from build123d import *

# Parameters (mm, degrees)
SKETCH1_R                       = 48.5
SKETCH1_R_2                     = 1.5
BOSS_EXTRUDE1_DEPTH             = 4
SKETCH2_R                       = 3.75
CUT_EXTRUDE1_DEPTH              = 1.5
BOSS_EXTRUDE2_START             = 4
SKETCH3_R                       = 9
BOSS_EXTRUDE2_DEPTH             = 14
CUT_EXTRUDE3_START              = 6
SKETCH4_R                       = 1.3
CUT_EXTRUDE3_DEPTH              = 91.444646155
BOSS_EXTRUDE3_DEPTH             = 9
BOSS_EXTRUDE3_DIRECTION_2_REACH = 108.638
CUT_EXTRUDE4_DEPTH              = 101.75311462
CUT_EXTRUDE4_DEPTH_BACK         = 101.75311462
FILLET1_R                       = 10
FILLET2_R                       = 2


with BuildPart() as part:
    # Sketch1 → Boss-Extrude1 (new body)
    with BuildSketch(Plane(origin=(0, 0, 0), x_dir=(1, 0, 0), z_dir=(0, 1, 0))):
        with Locations(Location((0, 0, 0), (0, 0, 270))):
            Circle(SKETCH1_R)
        with Locations(Location((0, 7.25, 0), (0, 0, 270))):
            Circle(SKETCH1_R_2, mode=Mode.SUBTRACT)
        with Locations(Location((0, -7.25, 0), (0, 0, 270))):
            Circle(SKETCH1_R_2, mode=Mode.SUBTRACT)
    extrude(amount=BOSS_EXTRUDE1_DEPTH)

    # Sketch2 → Cut-Extrude1 (cut)
    with BuildSketch(Plane.XZ):
        with Locations(Location((0, 0, 0), (0, 0, 270))):
            Circle(SKETCH2_R)
    extrude(amount=-CUT_EXTRUDE1_DEPTH, mode=Mode.SUBTRACT)

    # Sketch3 → Boss-Extrude2 (add)
    with BuildSketch(Plane(origin=(0, 0, 0), x_dir=(0, 0, -1), z_dir=(1, 0, 0)).offset(BOSS_EXTRUDE2_START)):
        with BuildLine():
            Line((30.34, 4), (-30.34, 4))
            Line((-30.34, 4), (-30.34, 11.86))
            ThreePointArc((-30.34, 11.86), (-28.924736696, 21.745164753), (-24.792654999, 30.836113728))
            Line((-24.792654999, 30.836113728), (-9.278105641, 55.104149989))
            ThreePointArc((-9.278105641, 55.104149989), (30.651097233, 62.12443475), (34.252718415, 21.743078098))
            ThreePointArc((34.252718415, 21.743078098), (31.352340729, 17.057138369), (30.34, 11.64))
            Line((30.34, 11.64), (30.34, 4))
        make_face()
        with Locations((13.91, 40.28)):
            Circle(SKETCH3_R, mode=Mode.SUBTRACT)
    extrude(amount=BOSS_EXTRUDE2_DEPTH)

    # Sketch4 → Cut-Extrude3 (cut, through all)
    with BuildSketch(Plane(origin=(0, 0, 0), x_dir=(0, 0, -1), z_dir=(1, 0, 0)).offset(CUT_EXTRUDE3_START)):
        Polygon((-15.259242405, 25.959242405), (13.732135624, 54.950620434), (28.581378029, 40.101378029), (-0.41, 11.11), align=None)
        with Locations(Location((-13.845028843, 19.595281374, 0), (0, 0, 180))):
            Circle(SKETCH4_R)
        with Locations(Location((-6.773961031, 12.524213562, 0), (0, 0, 180))):
            Circle(SKETCH4_R)
        with Locations(Location((20.096096654, 53.536406871, 0), (0, 0, 180))):
            Circle(SKETCH4_R)
        with Locations(Location((27.167164466, 46.465339059, 0), (0, 0, 180))):
            Circle(SKETCH4_R)
    extrude(amount=CUT_EXTRUDE3_DEPTH, mode=Mode.SUBTRACT)

    # Sketch5 → Boss-Extrude3 (add)
    with BuildSketch(Plane(origin=(18, 0, 0), x_dir=(0, 0, -1), z_dir=(1, 0, 0))):
        with BuildLine():
            Line((30.34, 4), (36.34, 4))
            Line((36.34, 4), (36.34, 11.64))
            ThreePointArc((36.34, 11.64), (36.947404437, 14.890283021), (38.687631049, 17.701846859))
            ThreePointArc((38.687631049, 17.701846859), (34.300821036, 66.886736311), (-14.333340667, 58.335960445))
            Line((-14.333340667, 58.335960445), (-29.847890025, 34.067924184))
            ThreePointArc((-29.847890025, 34.067924184), (-34.683704058, 23.428701186), (-36.34, 11.86))
            Line((-36.34, 11.86), (-36.34, 4))
            Line((-36.34, 4), (-30.34, 4))
            Line((-30.34, 4), (-30.34, 11.86))
            ThreePointArc((-30.34, 11.86), (-28.924736696, 21.745164753), (-24.792654999, 30.836113728))
            Line((-24.792654999, 30.836113728), (-14.162524076, 47.463886585))
            ThreePointArc((-14.162524076, 47.463886585), (-11.806963139, 51.339412511), (-9.278105641, 55.104149989))
            ThreePointArc((-9.278105641, 55.104149989), (30.651097233, 62.12443475), (34.252718415, 21.743078098))
            ThreePointArc((34.252718415, 21.743078098), (31.352340729, 17.057138369), (30.34, 11.64))
            Line((30.34, 11.64), (30.34, 4))
        make_face()
    extrude(amount=BOSS_EXTRUDE3_DEPTH)

    # Boss-Extrude3 direction 2: up to this face of the body (flat: up to its plane)
    boss_extrude3_direction_2_end = Plane(part.part.faces().sort_by_distance((4, 32.000889593, -6.762869766))[0])
    # Sketch5 → Boss-Extrude3 direction 2 (add, up to the picked face)
    with BuildSketch(Plane(origin=(18, 0, 0), x_dir=(0, 0, -1), z_dir=(1, 0, 0)), mode=Mode.PRIVATE) as boss_extrude3_direction_2_sk1:
        with BuildLine():
            Line((30.34, 4), (36.34, 4))
            Line((36.34, 4), (36.34, 11.64))
            ThreePointArc((36.34, 11.64), (36.947404437, 14.890283021), (38.687631049, 17.701846859))
            ThreePointArc((38.687631049, 17.701846859), (34.300821036, 66.886736311), (-14.333340667, 58.335960445))
            Line((-14.333340667, 58.335960445), (-29.847890025, 34.067924184))
            ThreePointArc((-29.847890025, 34.067924184), (-34.683704058, 23.428701186), (-36.34, 11.86))
            Line((-36.34, 11.86), (-36.34, 4))
            Line((-36.34, 4), (-30.34, 4))
            Line((-30.34, 4), (-30.34, 11.86))
            ThreePointArc((-30.34, 11.86), (-28.924736696, 21.745164753), (-24.792654999, 30.836113728))
            Line((-24.792654999, 30.836113728), (-14.162524076, 47.463886585))
            ThreePointArc((-14.162524076, 47.463886585), (-11.806963139, 51.339412511), (-9.278105641, 55.104149989))
            ThreePointArc((-9.278105641, 55.104149989), (30.651097233, 62.12443475), (34.252718415, 21.743078098))
            ThreePointArc((34.252718415, 21.743078098), (31.352340729, 17.057138369), (30.34, 11.64))
            Line((30.34, 11.64), (30.34, 4))
        make_face()
    boss_extrude3_direction_2_tool1 = split(extrude(boss_extrude3_direction_2_sk1.sketch, amount=-BOSS_EXTRUDE3_DIRECTION_2_REACH, mode=Mode.PRIVATE), bisect_by=boss_extrude3_direction_2_end, keep=Keep.BOTH, mode=Mode.PRIVATE)
    add(boss_extrude3_direction_2_tool1.solids().sort_by(Axis((18, 7.82, -31.430412), (-1, 0, 0)))[0])

    # Sketch6 → Cut-Extrude4 (cut, two sides: drawn at the far end of the back side and taken through both)
    with BuildSketch(Plane.XY.offset(-CUT_EXTRUDE4_DEPTH_BACK)):
        with BuildLine():
            Line((27, 73.801694463), (21, 73.801694463))
            ThreePointArc((21, 73.801694463), (22.52665425, 38.804454133), (26.5, 4))
            Line((26.5, 4), (27, 4))
            Line((27, 4), (27, 73.801694463))
        make_face()
    extrude(amount=CUT_EXTRUDE4_DEPTH + CUT_EXTRUDE4_DEPTH_BACK, mode=Mode.SUBTRACT)

    # Fillet1
    # the kernel refuses this fillet: 10 mm, written as the material it takes off along each edge
    with BuildSketch(Plane(origin=(4, 11.86, 36.34), x_dir=(0, 0, -1), z_dir=(0, -1, 0))) as fillet1_piece_1:
        with BuildLine():
            CenterArc((FILLET1_R, FILLET1_R), FILLET1_R, 180, 90)
            Line((0, FILLET1_R), (0, 0))
            Line((0, 0), (FILLET1_R, 0))
        make_face()
    extrude(amount=7.86, mode=Mode.SUBTRACT)
    with BuildSketch(Plane(origin=(4, 11.86, -4.89), x_dir=(0, 0.5386350760234976, 0.8425391711233141), z_dir=(0, 0.8425391711233141, -0.5386350760234976))) as fillet1_piece_2:
        with BuildLine():
            CenterArc((41.23 - FILLET1_R, FILLET1_R), FILLET1_R, 270, 90)
            Line((41.23, FILLET1_R), (41.23, 0))
            Line((41.23, 0), (41.23 - FILLET1_R, 0))
        make_face()
    revolve(axis=Axis((4, 11.86, -4.89), (1, 0, 0)), revolution_arc=32.590770812, mode=Mode.SUBTRACT)
    with BuildSketch(Plane(origin=(4, 58.335960445, 14.333340667), x_dir=(0, -0.5386350760234987, -0.8425391711233132), z_dir=(0, -0.8425391711233133, 0.5386350760234988))) as fillet1_piece_3:
        with BuildLine():
            CenterArc((FILLET1_R, FILLET1_R), FILLET1_R, 180, 90)
            Line((0, FILLET1_R), (0, 0))
            Line((0, 0), (FILLET1_R, 0))
        make_face()
    extrude(amount=28.803451629, mode=Mode.SUBTRACT)
    with BuildSketch(Plane(origin=(4, 40.28, -13.91), x_dir=(0, -0.6735385398377844, -0.7391521056948869), z_dir=(0, -0.7391521056948869, 0.6735385398377844))) as fillet1_piece_4:
        with BuildLine():
            CenterArc((33.521694463 - FILLET1_R, FILLET1_R), FILLET1_R, 270, 90)
            Line((33.521694463, FILLET1_R), (33.521694463, 0))
            Line((33.521694463, 0), (33.521694463 - FILLET1_R, 0))
        make_face()
    revolve(axis=Axis((4, 40.28, -13.91), (1, 0, 0)), revolution_arc=189.749991197, mode=Mode.SUBTRACT)
    with BuildSketch(Plane(origin=(4, 4, -36.34), x_dir=(0, 0, 1), z_dir=(0, 1, 0))) as fillet1_piece_5:
        with BuildLine():
            CenterArc((FILLET1_R, FILLET1_R), FILLET1_R, 180, 90)
            Line((0, FILLET1_R), (0, 0))
            Line((0, 0), (FILLET1_R, 0))
        make_face()
    extrude(amount=7.64, mode=Mode.SUBTRACT)
    with BuildSketch(Plane(origin=(4, 11.64, -45.34), x_dir=(0, 0.6735385398377856, 0.7391521056948859), z_dir=(0, 0.7391521056948859, -0.6735385398377856))) as fillet1_piece_6:
        with BuildLine():
            CenterArc((9 + FILLET1_R, FILLET1_R), FILLET1_R, 180, 90)
            Line((9, FILLET1_R), (9, 0))
            Line((9, 0), (9 + FILLET1_R, 0))
        make_face()
    revolve(axis=Axis((4, 11.64, -45.34), (1, 0, 0)), revolution_arc=42.340762009, mode=Mode.SUBTRACT)

    # Fillet2
    fillet2_edges = [part.edges().sort_by_distance(p)[0] for p in [
        (20.25, 4, -36.34),
        (20.25, 4, 36.34),
        (6.928932188, 4, 33.411067812),
        (4, 4, 0),
        (6.928932188, 4, -33.411067812),
    ]]
    fillet(fillet2_edges, radius=FILLET2_R)
    fillet2_2_edges = [part.edges().sort_by_distance(p)[0] for p in [
        (26.5, 4, -33.34),
    ]]
    fillet(fillet2_2_edges, radius=FILLET2_R)
    fillet2_3_edges = [part.edges().sort_by_distance(p)[0] for p in [
        (26.5, 4, 33.34),
    ]]
    fillet(fillet2_3_edges, radius=FILLET2_R)


solid = part.part
For this review, take the finished solid that the model builds, in its own axes (mm). A direction names the side the tool comes from. Give positions to 0.01 mm unless a question says otherwise; leave off trailing zeros. Loops run counter-clockwise (first coordinate to the right, second up) from the corner with the lowest first, then second, coordinate; pieces in that order, holes last.
Item 1: Take a section at A-A, the plane z = -7.25. Give the number of separate pieces and of enclosed holes in the cut face, and give its area (3 significant figures).
Item 2: Take a section at C-C, the plane x = -15. State the section outline as (y, z) points.
Item 3: Insertion check: pin 1 (4 mm diameter, centred on y = 55, z = 11, fed in from +X); pin 2 (6 mm diameter, centred on y = 50, z = -37.5, fed in from +X); pin 3 (1.8 mm diameter, centred on x = 17.5, y = 10, fed in from +Z). Each pin has a flat end and moves straight along its axis. Give the tip position at first contact, or say it passes through.
Item 4: Draft analysis for pull direction Y (two halves, no side actions). For faces 5 (the cylindrical face through (21.515, 54.988, 9.78)), 6 (the cylindrical face through (-43.028, 1.972, 22.38)), 7 (the flat face through (6, 54, -20)), state which applies: +Y half, -Y half, draft (parallel to the pull), parting line (faces both ways), or undercut.
Item 5: Take a section at D-D, the plane x = -39. State the section outline as (y, z) points, and give its area (3 significant figures).
Item 6: Tool access review of faces 1 (the cylindrical face through (7.01, 8.78, -33.49)), 2 (the flat face through (6, 28, -2)), 3 (the flat face through (0, 1.5, 0)), 4 (the flat face through (4, 29, -6)): name each direction out of +Z, -Z, +X, -X, +Y, -Y from which nothing blocks a thin tool from reaching the whole face with its end or side.
Item 7: For line 1 along X through (y, z) = (0.55, 0); line 2 along Z through (x, y) = (23, 10); line 3 along Y through (x, z) = (-27.5, -14), list the stretches that pass through material, from the lowest coordinate up.
Calculated:
1. separate pieces: 3
1. enclosed holes: 0
1. area: 957 mm2
2. outline: (0, -46.12) - (4, -46.12) - (4, 46.12) - (0, 46.12) - close
3. pin 1: stops at x = 21.61
3. pin 2: stops at x = 21.85
3. pin 3: stops at z = 36.34
4. face 5: +Y half
4. face 6: draft
4. face 7: undercut
5. outline: (0, -28.83) - (4, -28.83) - (4, 28.83) - (0, 28.83) - close
5. area: 231 mm2
6. face 1: -Z, -X
6. face 2: +X
6. face 3: -Y
6. face 4: +Z, -Z, -X, +Y
7. line 1: x = -48.5 to -3.75, 3.75 to 48.5
7. line 2: z = -36.34 to -30.34, 30.34 to 36.34
7. line 3: y = 0 to 4
